Geometry: final body of the model. Coordinates: model frame, mm. A direction names the side the tool comes from. Give positions to 0.01 mm unless a question says otherwise; leave off trailing zeros. Write each loop counter-clockwise with the first axis right and the second up, starting at its lowest first coordinate (ties: lowest second). Pieces come first, ordered by that corner, then holes.
Autodesk Inventor part; units mm, degrees
ref_plane "Work Plane1" through (-5, 30, -18.0278) normal (1, 0, 0) x (0, 0, 1)
ref_plane "YZ Plane" through (0, 0, 0) normal (1, 0, 0) x (0, 1, 0)
ref_plane "XZ Plane" through (0, 0, 0) normal (0, 1, 0) x (-1, 0, 0)
ref_plane "Work Plane1" through (-5, 30, -18.0278) normal (1, 0, 0) x (0, 0, 1)
sketch "Sketch2" plane through (-5, 30, -18.0278) normal (1, 0, 0) x (0, 0, 1)
  arc A0 (36.0555, 0) -> (48.0278, 11.9722) centre (18.0278, 30) ccw
  line L0 (48.0278, 11.9722) -> (48.0278, 48.0278)
  arc A1 (36.0555, 0) -> (48.0278, 11.9722) centre (18.0278, 30) ccw
  line L1 (48.0278, 48.0278) -> (48.0278, 11.9722)
  arc A2 (48.0278, 48.0278) -> (36.0555, 60) centre (18.0278, 30) ccw
  line L2 (48.0278, 48.0278) -> (48.0278, 60)
  line L3 (48.0278, 60) -> (-61.9722, 60)
  line L4 (-61.9722, 60) -> (-61.9722, 0)
  line L5 (0, 0) -> (36.0555, 0)
  line L6 (-61.9722, 0) -> (0, 0)
  line L7 (0, 0) -> (36.0555, 0)
extrude "Extrusion1" add sketch "Sketch2" along normal blind 26 and the other way blind 2
sketch "Sketch4" plane through (-7, -30, -80) normal (0, -1, 0) x (1, 0, 0)
  line L0 (28, 110) -> (28, 0)
  line L1 (0, 0) -> (0, 110)
  line L2 (28, 110) -> (0, 110)
  line L3 (0, 110) -> (0, 0)
  line L4 (0, 0) -> (28, 0)
  line L5 (28, 0) -> (28, 110)
  point P0 (7, 80)
extrude "Extrusion3" add sketch "Sketch4" along normal blind 1.028
sketch "Sketch5" plane through (21, 30, -18.0278) normal (1, 0, 0) x (0, 0, -1)
  arc A0 (-36.0555, 0) -> (-48.0278, -11.9722) centre (-18.0278, -30) ccw
  line L0 (-48.0278, -11.9722) -> (-48.0278, -61.028)
  line L1 (-48.0278, -11.9722) -> (-48.0278, -61.028)
  line L2 (61.9722, 0) -> (61.9722, -61.028)
  line L3 (-48.0278, -61.028) -> (61.9722, -61.028)
  line L4 (61.9722, -61.028) -> (61.9722, 0)
  line L5 (-36.0555, 0) -> (61.9722, 0)
  line L6 (61.9722, 0) -> (-36.0555, 0)
  arc A1 (-36.0555, 0) -> (-48.0278, -11.9722) centre (-18.0278, -30) ccw
  line L7 (55.9722, -55.028) -> (-42.0278, -55.028)
  line L8 (-42.0278, -55.028) -> (-42.0278, -13.7212)
  arc A2 (-34.3066, -6) -> (-42.0278, -13.7212) centre (-18.0278, -30) ccw
  line L9 (-34.3066, -6) -> (55.9722, -6)
  line L10 (55.9722, -6) -> (55.9722, -55.028)
  dimension "d11" = 6
extrude "Extrusion4" cut sketch "Sketch5" against normal blind 25 contours L7 L8 A2 L9 L10
sketch "Sketch6" plane through (-7, 30, -80) normal (-1, 0, 0) x (0, 0, 1)
  line L0 (0, 0) -> (98.0278, 0)
  line L1 (0, 0) -> (98.0278, 0)
  line L2 (0, -61.028) -> (110, -61.028)
  line L3 (110, -11.9722) -> (110, -61.028)
  line L4 (110, -61.028) -> (0, -61.028)
  line L5 (0, 0) -> (0, -61.028)
  line L6 (0, -61.028) -> (0, 0)
  line L7 (110, -11.9722) -> (110, -61.028)
  arc A0 (110, -11.9722) -> (98.0278, 0) centre (80, -30) ccw
  point P0 (80, -30)
extrude "Extrusion5" add sketch "Sketch6" along normal blind 10
sketch "Sketch7" plane through (-17, 30, -80) normal (-1, 0, 0) x (0, 0, 1)
  circle A0 centre (80, -30) radius 16.05
  dimension "d16" = 32.1
extrude "Extrusion6" cut sketch "Sketch7" against normal blind 13
fillet "Fillet1" radius 18.5 1 edges at (2, -31.028, 30)
properties part number "Tilt_Lid"
Item 1: Section B-B, the plane x = 4.5. Return the cut outline in (y, z), plus the area to 3 significant figures.
Found:
outline: (-31.03, -80) - (30, -80) - (30, 18.03) arc R35 ccw to (18.03, 30) - (-12.53, 30) arc R18.5 ccw to (-31.03, 11.5) - close; hole (-25.03, -74) - (24, -74) - (24, 16.28) arc R29 ccw to (16.28, 24) - (-25.03, 24) - close
area: 1,800 mm2
Item 2: Reachability of faces 5 (the face through (-4, 0, -24)), 6 (the face through (2, 3, 30)) from +Z, -Z, +X, -X, +Y, -Y: full face, straight path, thin tool, end or side. Return the list, or none.
Found:
face 5: +X
face 6: +Z, +X, -X, +Y, -Y
Item 3: Section A-A, the plane y = 0. Return the cut outline in (x, z).
Found:
outline: (-17, -80) - (21, -80) - (21, -74) - (-4, -74) - (-4, -16.05) - (-17, -16.05) - close; (-17, 16.05) - (-4, 16.05) - (-4, 24) - (21, 24) - (21, 30) - (-17, 30) - close
Item 4: Line query: L1, parallel to Y at x = 14, z = -42; L2, parallel to Y at x = -7.5, z = 0; L3, parallel to Z at x = -2, y = 6.5. Output: solid intervals per line, ascending.
Found:
L1: y = -31.03 to -25.03, 24 to 30
L2: y = -31.03 to -16.05, 16.05 to 30
L3: z = -80 to -74, 24 to 30
Item 5: Section D-D, the plane z = -48.5. Return the cut outline in (x, y).
Found:
outline: (-17, -31.03) - (21, -31.03) - (21, -25.03) - (-4, -25.03) - (-4, 24) - (21, 24) - (21, 30) - (-17, 30) - close
Item 6: Section C-C, the plane z = 0. Return the cut outline in (x, y), plus the area to 3 significant figures.
Found:
outline: (-17, -31.03) - (21, -31.03) - (21, -25.03) - (-4, -25.03) - (-4, -16.05) - (-17, -16.05) - close; (-17, 16.05) - (-4, 16.05) - (-4, 24) - (21, 24) - (21, 30) - (-17, 30) - close
area: 676 mm2
Item 7: Pull-direction query (Y, two-part tool) for faces 1 (the face through (2, -31.028, -35)), 2 (the face through (-10.591, -9.766, -12.737)), 3 (the face through (-17, 0, -26)), 4 (the face through (2, 30, -32)); classes: +Y half, -Y half, draft (parallel to the pull), parting line (faces both ways), or undercut.
Found:
face 1: -Y half
face 2: undercut
face 3: draft
face 4: +Y half
Item 8: Pin query (flat end, axial travel): pin 1 Ø2 at (x, y) = (-4, -17) entering from +Z. Return the tip coordinate at first contact, or that it passes through.
Found:
pin 1: stops at z = 29.67
